from build123d import *

# Parameters (mm, degrees)
ESQUISSE1_W             = 70
ESQUISSE1_H             = 36
ESQUISSE1_R             = 2.3
BOSS_EXTRU_1_DEPTH      = 7
ESQUISSE2_R             = 4
ENL_V_MAT_EXTRU_1_DEPTH = 4
BOSS_EXTRU_2_DEPTH      = 70


with BuildPart() as part:
    # Esquisse1 → Boss.-Extru.1 (new body)
    with BuildSketch(Plane.XY):
        with Locations((35, 18)):
            Rectangle(ESQUISSE1_W, ESQUISSE1_H)
        with Locations((5, 25.5)):
            Circle(ESQUISSE1_R, mode=Mode.SUBTRACT)
        with Locations((5, 10.5)):
            Circle(ESQUISSE1_R, mode=Mode.SUBTRACT)
        with Locations((23.125, 25.5)):
            Circle(ESQUISSE1_R, mode=Mode.SUBTRACT)
        with Locations((23.125, 10.5)):
            Circle(ESQUISSE1_R, mode=Mode.SUBTRACT)
        with Locations((41.25, 25.5)):
            Circle(ESQUISSE1_R, mode=Mode.SUBTRACT)
        with Locations((41.25, 10.5)):
            Circle(ESQUISSE1_R, mode=Mode.SUBTRACT)
        with Locations((59.375, 25.5)):
            Circle(ESQUISSE1_R, mode=Mode.SUBTRACT)
        with Locations((59.375, 10.5)):
            Circle(ESQUISSE1_R, mode=Mode.SUBTRACT)
    extrude(amount=BOSS_EXTRU_1_DEPTH)

    # Esquisse2 → Enlèv. mat.-Extru.1 (cut)
    with BuildSketch(Plane(origin=(0, 0, 0), x_dir=(-1, 0, 0), z_dir=(0, 0, -1))):
        with Locations((-59.375, 25.5)):
            Circle(ESQUISSE2_R)
        with Locations((-41.25, 25.5)):
            Circle(ESQUISSE2_R)
        with Locations((-23.125, 25.5)):
            Circle(ESQUISSE2_R)
        with Locations((-5, 25.5)):
            Circle(ESQUISSE2_R)
        with Locations((-5, 10.5)):
            Circle(ESQUISSE2_R)
        with Locations((-23.125, 10.5)):
            Circle(ESQUISSE2_R)
        with Locations((-41.25, 10.5)):
            Circle(ESQUISSE2_R)
        with Locations((-59.375, 10.5)):
            Circle(ESQUISSE2_R)
    extrude(amount=-ENL_V_MAT_EXTRU_1_DEPTH, mode=Mode.SUBTRACT)

    # Esquisse3 → Boss.-Extru.2 (add)
    with BuildSketch(Plane(origin=(70, 0, 0), x_dir=(0, 0, -1), z_dir=(1, 0, 0))):
        Polygon((-41.167503398, 59.077731941), (0, 36), (-7, 36), (-44.587704831, 49.680805733), align=None)
        Polygon((-44.587704831, -13.680805733), (-41.167503398, -23.077731941), (0, 0), (-7, 0), align=None)
    extrude(amount=-BOSS_EXTRU_2_DEPTH)


solid = part.part
Read the model definition and answer for the solid it produces. Units are mm, in the model's axes. A direction names the side the tool comes from. Give positions to 0.01 mm unless a question says otherwise; leave off trailing zeros. Write each loop counter-clockwise with the first axis right and the second up, starting at its lowest first coordinate (ties: lowest second). Pieces come first, ordered by that corner, then holes. Notation, with made-up numbers: (13.25, 11.5) -> (51.25, 11.5) arc R19 cw to (51.25, 44.5) -> close; hole circle Ø9 at (2, 80). An arc over 180 degrees is marked (long way). Answer as a JSON object with one key per item and string values. Group by question number.
1) A tool of negligible diameter and unlimited length cuts with its end or side. For faces 4 (the cylindrical face through (26.073, 13.203, 1.972)), 5 (the flat face through (35.49, -6.745, 25.531)), 6 (the flat face through (35.49, 47.7, 20.87)), from which of +Z, -Z, +X, -X, +Y, -Y can it reach the whole face along a straight path? Write none if from no direction.
2) Consider L1, parallel to X at y = 10, z = 5 (3 decimals); L2, parallel to X at y = 25.5, z = 6.3 (3 decimals); L3, parallel to Y at x = 41, z = 6. Determine where each line is inside the solid, lowest interval first. Write a range as from..to.
3) Find section A-A (z = 14). Write down the section's boundary in (x, y).
4) Find section C-C (y = 25.5). Count the separate pieces of the cut face and the enclosed holes in it, and give its area (3 significant figures).
5) Find section D-D (x = 12). Write down the section's boundary in (y, z).
6) The mould has two halves that part along X. Classify faces 1 (the flat face through (35.49, -11.7, 20.87)), 2 (the cylindrical face through (61.57, 11.19, 5.48)), 3 (the flat face through (0, 18, 6)): +X half, -X half, draft (parallel to the pull), parting line (faces both ways), or undercut.
7) Each of these flat-tipped pins is pushed along its axis until it touches: P1, Ø2.5, axis at x = 58.5, y = 26.5, coming from the -Z side; P2, Ø4, axis at x = 59.375, y = 10.5, coming from the +Z side; P3, Ø13, axis at x = 59.375, y = 10.5, coming from the +Z side; P4, Ø12, axis at x = 32, z = 33.5, coming from the +Y side. Where does it stop, or does it pass through?
8) Find section B-B (x = 5). Write down the section's boundary in (y, z).
Values follow:
{
 "1": {"face 4": "-Z", "face 5": "+Z, +X, -X", "face 6": "-Z, +X, -X, +Y"},
 "2": {"L1": "x = 0..2.755, 7.245..20.88, 25.37..39.005, 43.495..57.13, 61.62..70", "L2": "x = 0..2.7, 7.3..20.825, 25.425..38.95, 43.55..57.075, 61.675..70", "L3": "y = -3.36..8.21, 12.79..23.21, 27.79..39.36"},
 "3": {"outline": "(0, -7.85) -> (70, -7.85) -> (70, -2.55) -> (0, -2.55) -> close; (0, 38.55) -> (70, 38.55) -> (70, 43.85) -> (0, 43.85) -> close"},
 "4": {"separate pieces": "5", "enclosed holes": "0", "area": "307 mm2"},
 "5": {"outline": "(-23.08, 41.17) -> (0, 0) -> (36, 0) -> (59.08, 41.17) -> (49.68, 44.59) -> (36, 7) -> (0, 7) -> (-13.68, 44.59) -> close"},
 "6": {"face 1": "draft", "face 2": "undercut", "face 3": "-X half"},
 "7": {"P1": "stops at z = 4", "P2": "passes through", "P3": "stops at z = 7", "P4": "stops at y = 58.14"},
 "8": {"outline": "(-23.08, 41.17) -> (0, 0) -> (6.5, 0) -> (6.5, 4) -> (8.2, 4) -> (8.2, 7) -> (0, 7) -> (-13.68, 44.59) -> close; (12.8, 4) -> (14.5, 4) -> (14.5, 0) -> (21.5, 0) -> (21.5, 4) -> (23.2, 4) -> (23.2, 7) -> (12.8, 7) -> close; (27.8, 4) -> (29.5, 4) -> (29.5, 0) -> (36, 0) -> (59.08, 41.17) -> (49.68, 44.59) -> (36, 7) -> (27.8, 7) -> close"}
}
